The listing builds one solid part. Answer for the finished solid, in the listing's coordinates (mm). A direction names the side the tool comes from. Coordinates: 2 decimals unless noted, no trailing zeros. Loops run counter-clockwise (first coordinate to the right, second up) from the corner with the lowest first, then second, coordinate; pieces in that order, holes last. Notation, with made-up numbers: M 15.5,16.5 L 71.5,16.5 A26 cw 71.5,39.5 Z; hole C -19.75,31.25 d11. An arc over 180 degrees is marked long. Return JSON: item names as keys, results as strings. Group by question number.
1. Section C-C (x = -3) is taken. Write down the section's boundary in (y, z), then the cut area to 3 significant figures.
2. Given P1, Ø8, axis at y = -12, z = 20, coming from the +X side; P2, Ø2, axis at x = 18, y = -23, coming from the +Z side; P3, Ø4, axis at x = -3.5, z = 15.5, coming from the -Y side, each flat-ended and moving along its own axis, determine where each tip first touches the part or whether it passes through.
3. Which of the six approach directions +Z, -Z, +X, -X, +Y, -Y give full straight-line access (tool end or side, diameter ignored) to faces 1 (the face through (43.138, -7, 18)), 2 (the face through (43.138, -17, -5)), 3 (the face through (-39, -32.791, -5))?
4. Section D-D (x = 34.5) is taken. Write down the section's boundary in (y, z).
5. Straight lines are drawn through the part: L1, parallel to Z at x = 4.5, y = -2.5; L2, parallel to X at y = -15, z = -7; L3, parallel to Z at x = 6, y = -17.5. For each, find the intervals that lie inside material, in ascending order. Write a range as from..to.
6. Section B-B (z = -5.5) is taken. Write down the section's boundary in (x, y), then the cut area to 3 significant figures.
7. The mould has two halves that part along Y. Classify faces 4 (the face through (-5.96, -15.25, 6.39)), 5 (the face through (-1, -16, 0)), 6 (the face through (-25.736, -16.625, -4.884)): pulls with the +Y half, pulls with the -Y half, needs draft (parallel to the pull), parting line crosses it, or undercut.
```python
from build123d import *

# Parameters (mm, degrees)
F1_DEPTH = 13.462
F2_W     = 89.7744297981
F2_H     = 33.0824591219
F3_DEPTH = 12.954
F4_R     = 7.6951725226
F5_DEPTH = 63.5
F6_W     = 14.5737677813
F6_H     = 32.7909812331
F6_W_2   = 13.6993471533
F6_H_2   = 33.3739332855
F7_DEPTH = 9.906


with BuildPart() as f1:
    # F0 (on Front) → F1 (new body)
    with BuildSketch(Plane.XZ):
        Polygon((-27.1072126925, 37.1631160378), (-46.0531152785, 22.5893463939), (-46.0531152785, 0), (43.1383624673, 0), (43.1383624673, 22.5893463939), (27.1072126925, 37.1631160378), align=None)
    extrude(amount=F1_DEPTH)

    # F2 (on Top) → F3 (join)
    with BuildSketch(Plane.XY):
        with Locations((-1.4573782682, -16.541229561)):
            Rectangle(F2_W, F2_H)
    extrude(amount=F3_DEPTH)

    # F4 (on Top) → F5 (cut)
    with BuildSketch(Plane.XY):
        with Locations((-4.9550817348, -22.8808205575)):
            Circle(F4_R)
    extrude(amount=F5_DEPTH, mode=Mode.SUBTRACT)

    # F6 (on Top) → F7 (join)
    with BuildSketch(Plane.XY):
        with Locations((-39.0577055514, -16.3954906166)):
            Rectangle(F6_W, F6_H)
        Polygon((-31.7708216608, 0), (-31.7708216608, -32.7909812331), (-19.5288527757, 0), align=None)
        with Locations((36.2886888906, -16.6869666427)):
            Rectangle(F6_W_2, F6_H_2)
        Polygon((16.6140999645, 0), (29.439015314, -33.3739332855), (29.439015314, 0), align=None)
    extrude(amount=-F7_DEPTH)


solid = f1.part
```
Worked out:
{
 "1": {"outline": "M -33.08,0 L -30.32,0 L -30.32,12.95 L -33.08,12.95 Z; M -15.44,0 L 0,0 L 0,37.16 L -13.46,37.16 L -13.46,12.95 L -15.44,12.95 Z", "area": "562 mm^2"},
 "2": {"P1": "x = 43.14", "P2": "z = 12.95", "P3": "y = -13.46"},
 "3": {"face 1": "+Z, +X, +Y, -Y", "face 2": "-Z, +X, +Y, -Y", "face 3": "-Z, -X, -Y"},
 "4": {"outline": "M -33.37,-9.91 L 0,-9.91 L 0,30.44 L -13.46,30.44 L -13.46,12.95 L -33.08,12.95 L -33.08,0 L -33.37,0 Z"},
 "5": {"L1": "0..37.16", "L2": "-46.34..-25.13, 22.38..43.14", "L3": "0..12.95"},
 "6": {"outline": "M -46.34,-32.79 L -31.77,-32.79 L -19.53,0 L -46.34,0 Z; M 16.61,0 L 29.44,-33.37 L 43.14,-33.37 L 43.14,0 Z", "area": "1,350 mm^2"},
 "7": {"face 4": "undercut", "face 5": "needs draft", "face 6": "pulls with the -Y half"}
}
